from build123d import *

# Parameters (mm, degrees)
F0_W     = 279.4
F0_H     = 279.4
F1_DEPTH = 6.35
F5_R     = 2.2225
F7_R     = 1.905
F8_DEPTH = 5.08


with BuildPart() as f1:
    # F0 (on Top) → F1 (new body)
    with BuildSketch(Plane.XY):
        with Locations((139.7, 139.7)):
            Rectangle(F0_W, F0_H)
    extrude(amount=F1_DEPTH)

    # F6: sweep along a path in F3
    with BuildLine(Plane.XZ.offset(-139.7)) as f6_path:
        CenterArc((139.7, 19.05), 12.7, 0, 360)
    # F5 (on offset) → F6 (sweep)
    with BuildSketch(Plane.YZ.offset(139.7)):
        with Locations((139.7, 6.35)):
            Circle(F5_R)
    sweep(path=f6_path.line)

    # F7 (on face) → F8 (cut)
    with BuildSketch(Plane(origin=(0, 0, 0), x_dir=(1, 0, 0), z_dir=(0, 0, -1))):
        with Locations((38.1, -38.1)):
            Circle(F7_R)
        with Locations((88.9, -38.1)):
            Circle(F7_R)
        with Locations((139.7, -38.1)):
            Circle(F7_R)
        with Locations((241.3, -38.1)):
            Circle(F7_R)
        with Locations((190.5, -38.1)):
            Circle(F7_R)
        with Locations((38.1, -88.9)):
            Circle(F7_R)
        with Locations((88.9, -88.9)):
            Circle(F7_R)
        with Locations((139.7, -88.9)):
            Circle(F7_R)
        with Locations((190.5, -88.9)):
            Circle(F7_R)
        with Locations((241.3, -88.9)):
            Circle(F7_R)
        with Locations((38.1, -139.7)):
            Circle(F7_R)
        with Locations((88.9, -139.7)):
            Circle(F7_R)
        with Locations((139.7, -139.7)):
            Circle(F7_R)
        with Locations((190.5, -139.7)):
            Circle(F7_R)
        with Locations((241.3, -139.7)):
            Circle(F7_R)
        with Locations((241.3, -190.5)):
            Circle(F7_R)
        with Locations((190.5, -190.5)):
            Circle(F7_R)
        with Locations((139.7, -190.5)):
            Circle(F7_R)
        with Locations((88.9, -190.5)):
            Circle(F7_R)
        with Locations((38.1, -190.5)):
            Circle(F7_R)
        with Locations((38.1, -241.3)):
            Circle(F7_R)
        with Locations((88.9, -241.3)):
            Circle(F7_R)
        with Locations((139.7, -241.3)):
            Circle(F7_R)
        with Locations((190.5, -241.3)):
            Circle(F7_R)
        with Locations((241.3, -241.3)):
            Circle(F7_R)
    extrude(amount=-F8_DEPTH, mode=Mode.SUBTRACT)


solid = f1.part
Build history of the part. All positions in model axes, mm. Give positions to 0.01 mm unless a question says otherwise; leave off trailing zeros. Order: outer loops, then holes, each group sorted by start corner. A loop starts at its lowest first (then second) coordinate and runs counter-clockwise, first axis right, second up. Notation, with made-up numbers: M 67.5,49 L 96.5,49 A29 ccw 96.5,81 Z; hole C -7,-8.5 d5. An arc over 180 degrees is marked long. Use one line per item in the form item = value.
Q1. Wall check: probe 1 along Y at (x, z) = (38, 2); probe 2 along X at (y, z) = (241, 2); probe 3 along X at (y, z) = (139, 1). Give the ranges that are in metal, low to high.
Conclusion:
probe_1 = 0 to 36.2, 40 to 87, 90.8 to 137.8, 141.6 to 188.6, 192.4 to 239.4, 243.2 to 279.4
probe_2 = 0 to 36.22, 39.98 to 87.02, 90.78 to 137.82, 141.58 to 188.62, 192.38 to 239.42, 243.18 to 279.4
probe_3 = 0 to 36.33, 39.87 to 87.13, 90.67 to 137.93, 141.47 to 188.73, 192.27 to 239.53, 243.07 to 279.4
Q2. Pin check, flat tips, straight feed: P1, Ø6, axis at x = 88.9, y = 38.1, coming from the +Z side; P2, Ø1.9, axis at x = 38.5, y = 37.5, coming from the -Z side; P3, Ø5, axis at x = 190.5, y = 190.5, coming from the +Z side; P4, Ø8, axis at x = 136.5, z = 14, coming from the -Y side. Stop position of each tip, or through.
Conclusion:
P1 = 6.35
P2 = 5.08
P3 = 6.35
P4 = through
Q3. Slice it at A-A, the plane x = 235. Write the cut outline in (y, z), and give its area (3 significant figures).
Conclusion:
outline = M 0,0 L 279.4,0 L 279.4,6.35 L 0,6.35 Z
area = 1,770 mm2
